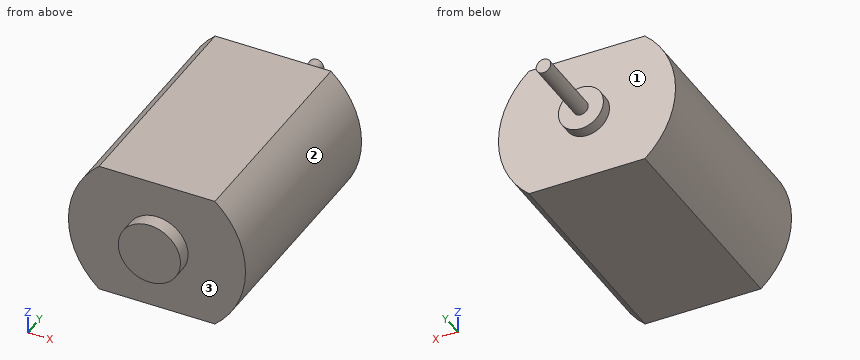
from build123d import *

# Parameters (mm, degrees)
BOSS_EXTRUDE1_DEPTH = 30.5
SKETCH3_R           = 3.075
BOSS_EXTRUDE2_DEPTH = 1.6
SKETCH4_R           = 1
BOSS_EXTRUDE3_DEPTH = 9.85
SKETCH5_R           = 4.25
BOSS_EXTRUDE4_DEPTH = 2


with BuildPart() as part:
    # Sketch2 → Boss-Extrude1 (new body)
    with BuildSketch(Plane(origin=(0, 0, 0), x_dir=(1, 0, 0), z_dir=(0, 1, 0))):
        with BuildLine():
            Line((-7.917543811, 9.15), (7.917543811, 9.15))
            ThreePointArc((7.917543811, 9.15), (12.1, 0), (7.917543811, -9.15))
            Line((7.917543811, -9.15), (-7.917543811, -9.15))
            ThreePointArc((-7.917543811, -9.15), (-12.1, 0), (-7.917543811, 9.15))
        make_face()
    extrude(amount=BOSS_EXTRUDE1_DEPTH)

    # Sketch3 → Boss-Extrude2 (add)
    with BuildSketch(Plane(origin=(0, 30.5, 0), x_dir=(1, 0, 0), z_dir=(0, 1, 0))):
        with Locations(Location((0, 0, 0), (0, 0, 270))):
            Circle(SKETCH3_R)
    extrude(amount=BOSS_EXTRUDE2_DEPTH)

    # Sketch4 → Boss-Extrude3 (add)
    with BuildSketch(Plane(origin=(0, 32.1, 0), x_dir=(1, 0, 0), z_dir=(0, 1, 0))):
        with Locations(Location((0, 0, 0), (0, 0, 270))):
            Circle(SKETCH4_R)
    extrude(amount=BOSS_EXTRUDE3_DEPTH)

    # Sketch5 → Boss-Extrude4 (add)
    with BuildSketch(Plane.XZ):
        with Locations(Location((0, 0, 0), (0, 0, 270))):
            Circle(SKETCH5_R)
    extrude(amount=BOSS_EXTRUDE4_DEPTH)


solid = part.part
Read the model definition and answer for the solid it produces. Units are mm, in the model's axes. Face numbers are marked on the shaded views. A direction names the side the tool comes from. Coordinates: 2 decimals unless noted, no trailing zeros. Order: outer loops, then holes, each group sorted by start corner. A loop starts at its lowest first (then second) coordinate and runs counter-clockwise, first axis right, second up. Notation, with made-up numbers: (-16, 28.25) -> (-12, 28.25) arc R28 ccw to (-12, 54.25) -> close; hole circle Ø2 at (37, -0.5). An arc over 180 degrees is marked (long way). Answer as a JSON object with one key per item and string values.
1) Each of these flat-tipped pins is pushed along its axis until it touches: pin 1 (8 mm diameter, centred on x = 7, z = -2, fed in from -Y); pin 2 (5.5 mm diameter, centred on x = -4, z = 0, fed in from +Y); pin 3 (2 mm diameter, centred on y = 6.5, z = -7, fed in from +X); pin 4 (3 mm diameter, centred on x = 6, z = -4, fed in from +Y). Where does it stop, or does it pass through?
Model answer:
{"pin 1": "stops at y = -2", "pin 2": "stops at y = 32.1", "pin 3": "stops at x = 10.51", "pin 4": "stops at y = 30.5"}
2) A tool of negligible diameter and unlimited length cuts with its end or side. For the marked faces 1, 2 and 3, from which of +Z, -Z, +X, -X, +Y, -Y can it reach the whole face along a straight path? Write none if from no direction.
Model answer:
{"face 1": "+Y", "face 2": "+X, +Y, -Y", "face 3": "-Y"}
3) A cutting plane is placed at A-A, the plane z = 0. Determine the outline of the cut face in (x, y) (3 decimals), plus the area to 3 significant figures.
Model answer:
{"outline": "(-12.1, 0) -> (-4.25, 0) -> (-4.25, -2) -> (4.25, -2) -> (4.25, 0) -> (12.1, 0) -> (12.1, 30.5) -> (3.075, 30.5) -> (3.075, 32.1) -> (1, 32.1) -> (1, 41.95) -> (-1, 41.95) -> (-1, 32.1) -> (-3.075, 32.1) -> (-3.075, 30.5) -> (-12.1, 30.5) -> close", "area": "785 mm²"}
4) A cutting plane is placed at C-C, the plane y = 18.5. Determine the outline of the cut face in (x, z), plus the area to 3 significant figures.
Model answer:
{"outline": "(-7.92, -9.15) -> (7.92, -9.15) arc R12.1 ccw to (7.92, 9.15) -> (-7.92, 9.15) arc R12.1 ccw to start", "area": "396 mm²"}
5) A cutting plane is placed at B-B, the plane x = 3.75. Determine the outline of the cut face in (y, z), plus the area to 3 significant figures.
Model answer:
{"outline": "(-2, -2) -> (0, -2) -> (0, -9.15) -> (30.5, -9.15) -> (30.5, 9.15) -> (0, 9.15) -> (0, 2) -> (-2, 2) -> close", "area": "566 mm²"}
6) A cutting plane is placed at D-D, the plane x = 0. Determine the outline of the cut face in (y, z) (3 decimals), plus the area to 3 significant figures.
Model answer:
{"outline": "(-2, -4.25) -> (0, -4.25) -> (0, -9.15) -> (30.5, -9.15) -> (30.5, -3.075) -> (32.1, -3.075) -> (32.1, -1) -> (41.95, -1) -> (41.95, 1) -> (32.1, 1) -> (32.1, 3.075) -> (30.5, 3.075) -> (30.5, 9.15) -> (0, 9.15) -> (0, 4.25) -> (-2, 4.25) -> close", "area": "605 mm²"}
7) Consider line 1 along Y through (x, z) = (-10, -4); line 2 along X through (y, z) = (24.5, 0.5); line 3 along Y through (x, z) = (-1.5, 0). Determine where each line is inside the solid, lowest interval first. Write a range as from..to.
Model answer:
{"line 1": "y = 0..30.5", "line 2": "x = -12.09..12.09", "line 3": "y = -2..32.1"}
